CAD build for the part. Positions are in the model's coordinates, mm. A direction names the side the tool comes from. Give positions to 0.01 mm unless a question says otherwise; leave off trailing zeros. Write each loop counter-clockwise with the first axis right and the second up, starting at its lowest first coordinate (ties: lowest second). Pieces come first, ordered by that corner, then holes. Notation, with made-up numbers: (63, 44.25) -> (82, 44.25) arc R25 cw to (82, 81.25) -> close; hole circle Ø5 at (25, 26.5). An arc over 180 degrees is marked (long way). Answer as a JSON object with one key per item and string values.
Autodesk Inventor part; units mm, degrees
ref_plane "YZ Plane" through (0, 0, 0) normal (1, 0, 0) x (0, 1, 0)
ref_plane "XZ Plane" through (0, 0, 0) normal (0, 1, 0) x (-1, 0, 0)
ref_plane "XY Plane" through (0, 0, 0) normal (0, 0, 1) x (1, 0, 0)
sketch "Sketch1" plane through (0, 0, 0) normal (0, 0, 1) x (1, 0, 0)
  arc A0 (-74.2, 0) -> (74.2, 0) centre (0, 603.0231) ccw construction
  arc A1 (-76.3128, -17.1705) -> (76.3128, -17.1705) centre (0, 603.0231) ccw
  arc A2 (-72.0872, 17.1705) -> (72.0872, 17.1705) centre (0, 603.0231) ccw
  arc A3 (-72.0872, 17.1705) -> (-76.3128, -17.1705) centre (-74.2, 0) ccw
  arc A4 (76.3128, -17.1705) -> (72.0872, 17.1705) centre (74.2, 0) ccw
  line L0 (-159.9202, 0) -> (186.0645, 0) construction
  line L1 (0, 827.4607) -> (0, -503.7998) construction
  line L2 (74.2, 0) -> (74.2, 0) construction
  line L3 (74.2, 0) -> (91.3705, 2.1128) construction
  line L4 (74.2, 0) -> (72.0872, 17.1705) construction
  circle A5 centre (74.2, 0) radius 8 construction
  circle A6 centre (73.223, 7.9401) radius 1.15
  circle A7 centre (66.2599, -0.977) radius 1.15
  circle A8 centre (75.177, -7.9401) radius 1.15
  circle A9 centre (82.1401, 0.977) radius 1.15
  circle A10 centre (-74.2, 0) radius 2.15
  circle A11 centre (-24.7333, -4.0442) radius 2.15
  circle A12 centre (24.7333, -4.0442) radius 2.15
  point P0 (0, 0)
  dimension "d3" = 16
  dimension "d0" = 148.4
  dimension "d1" = 34.6
  dimension "d2" = 603.0231
  dimension "d4" = 2.3
  dimension "d7" = 360
  dimension "d9" = 49.4667
  dimension "d10" = 24.7333
  dimension "d11" = 4.3
  dimension "d12" = 4.3
  dimension "d13" = 4.3
  dimension "d46" = 7.015
extrude "Extrusion1" add sketch "Sketch1" along normal blind 6 contours A3 A2 A4 A1 | A6 | A7 | A8 | A9
sketch "Sketch2" plane through (0, 0, 6) normal (0, 0, 1) x (1, 0, 0)
  circle A0 centre (-24.7333, -4.0442) radius 2.15
  line L0 (-21.0756, -6.0794) -> (-24.667, -8.2295)
  line L1 (-24.667, -8.2295) -> (-28.3247, -6.1943)
  line L2 (-28.3247, -6.1943) -> (-28.3911, -2.0091)
  line L3 (-28.3911, -2.0091) -> (-24.7997, 0.141)
  line L4 (-24.7997, 0.141) -> (-21.142, -1.8941)
  line L5 (-21.142, -1.8941) -> (-21.0756, -6.0794)
  circle A1 centre (24.7333, -4.0442) radius 2.15
  line L6 (21.2567, -6.3753) -> (20.9762, -2.199)
  line L7 (20.9762, -2.199) -> (24.4529, 0.1321)
  line L8 (24.4529, 0.1321) -> (28.2099, -1.7132)
  line L9 (28.2099, -1.7132) -> (28.4904, -5.8895)
  line L10 (28.4904, -5.8895) -> (25.0138, -8.2206)
  line L11 (25.0138, -8.2206) -> (21.2567, -6.3753)
  point P0 (0, 0)
  dimension "d16" = 7.25
  dimension "d22" = 7.25
extrude "Extrusion2" cut sketch "Sketch2" against normal blind 2
chamfer "Chamfer1" distance 2 angle 45 2 edges at (-26.8833, -4.0442, 4) (22.5833, -4.0442, 4)
sketch "Sketch4" plane through (0, 0, 0) normal (0, 0, -1) x (-1, 0, 0)
  line L0 (-73.223, 7.9401) -> (-75.177, -7.9401) construction
  circle A0 centre (-74.2, 0) radius 8 construction
  line L1 (-66.2, 0) -> (-95.5949, 0) construction
  line L2 (-66.2, 0) -> (0, 0) construction
  circle A1 centre (-75.177, -7.9401) radius 1.15 construction
  circle A2 centre (-66.2599, -0.977) radius 1.15 construction
  circle A3 centre (-73.223, 7.9401) radius 1.15 construction
  circle A4 centre (-82.1401, 0.977) radius 1.15 construction
  dimension "d28" = 82.985
  dimension "d29" = 16
  dimension "d30" = 2.3
  dimension "d31" = 74.2
  dimension "d34" = 360
hole "Hole1" at (75.177, -7.9401, 0) at (82.1401, 0.977, 0) at (73.223, 7.9401, 0) at (66.2599, -0.977, 0) direction (0, 0, 1) diameter 2.3 end through all counterbore diameter 4.5 counterbore depth 2
chamfer "Chamfer2" distance 1.1 angle 45 4 edges at (75.177, -9.0901, 2) (82.1401, -0.173, 2) (66.2599, -2.127, 2) (73.223, 6.7901, 2)
equation "\"d22\" = d16"
properties part number "Arm 12X"
1) Slice it at B-B (x = 33). List the corners of the cut face in (y, z).
Model answer:
{"outline": "(-20.98, 0) -> (13.68, 0) -> (13.68, 6) -> (-20.98, 6) -> close"}
2) 3-axis set-ups, long thin cutter, end or side, ignore diameter. For faces 1 (the cylindrical face through (77.373, -8.428, 1.014)), 2 (the cylindrical face through (22.585, -4.139, 0.986)): which of +Z, -Z, +X, -X, +Y, -Y reach the whole face in a straight line?
Model answer:
{"face 1": "-Z", "face 2": "+Z, -Z"}
3) Wall check: probe 1 along Y at (x, z) = (74, 0.6); probe 2 along X at (y, z) = (1.5, 0.4); probe 3 along X at (y, z) = (-4, 1.7). Give the ranges that are in metal, low to high.
Model answer:
{"probe 1": "y = -17.45 to -9.86, -6.02 to 5.83, 10.05 to 17.3", "probe 2": "x = -91.43 to -75.74, -72.66 to 79.95, 84.33 to 91.43", "probe 3": "x = -91.03 to -26.88, -22.58 to 22.58, 26.88 to 91.03"}
4) Pin check, flat tips, straight feed: pin 1 (2 mm diameter, centred on y = 8, z = 4.5, fed in from +X); pin 2 (1.3 mm diameter, centred on x = 75, y = -7, fed in from -Z); pin 3 (2 mm diameter, centred on x = 73.5, y = 8, fed in from -Z); pin 4 (1.8 mm diameter, centred on x = 66.26, y = -0.98, fed in from +Z). Stop position of each tip, or through.
Model answer:
{"pin 1": "stops at x = 90.02", "pin 2": "stops at z = 2.64", "pin 3": "stops at z = 2.97", "pin 4": "passes through"}
5) Slice it at C-C (y = -13). List the corners of the cut face in (x, z), then the cut area to 3 significant figures.
Model answer:
{"outline": "(-85.61, 0) -> (85.61, 0) -> (85.61, 6) -> (-85.61, 6) -> close", "area": "1,030 mm2"}
6) Mould opens along Y. For faces 3 (the cylindrical face through (1.012, 12.753, 2.958)), 4 (the flat face through (-1, -2, 6)), 5 (the conical face through (-27.01, -3.94, 2.13)) say: released by +Y, released by -Y, zero draft, split by the parting line, or undercut.
Model answer:
{"face 3": "released by +Y", "face 4": "zero draft", "face 5": "undercut"}
7) Slice it at A-A (x = -74.2). List the corners of the cut face in (y, z).
Model answer:
{"outline": "(-17.43, 0) -> (-2.15, 0) -> (-2.15, 6) -> (-17.43, 6) -> close; (2.15, 0) -> (17.3, 0) -> (17.3, 6) -> (2.15, 6) -> close"}
